CAD build for the part. Positions are in the model's coordinates, mm. A direction names the side the tool comes from. Coordinates: 2 decimals unless noted, no trailing zeros. Loops run counter-clockwise (first coordinate to the right, second up) from the corner with the lowest first, then second, coordinate; pieces in that order, holes last. Notation, with made-up numbers: (25.5, -33.5) -> (66.5, -33.5) arc R29 cw to (66.5, -3.5) -> close; hole circle Ø1 at (33.5, 13.25). An arc over 180 degrees is marked (long way). Write each question's results on one line, items separated by ' | '.
from build123d import *

# Parameters (mm, degrees)
BOSS_EXTRUDE1_DEPTH   = 1.5875
F_4_CLEARANCE_HOLE1_D = 2.9464


with BuildPart() as part:
    # Sketch2 → Boss-Extrude1 (new body)
    with BuildSketch(Plane.XY):
        Polygon((-2.1971, 2.8575), (2.1971, 2.8575), (2.1971, -2.8575), (7.9375, -2.8575), (7.9375, 6.6675), (-7.9375, 6.6675), (-7.9375, -2.8575), (-2.1971, -2.8575), align=None)
    extrude(amount=BOSS_EXTRUDE1_DEPTH)

    # #4 Clearance Hole1 (through all)
    with Locations(Plane.XY.offset(1.5875)):
        with Locations((-5.0673, 1.905), (5.0673, 1.905)):
            Hole(F_4_CLEARANCE_HOLE1_D / 2)


solid = part.part
1) Two-plate mould, pull along X, no slides. Class faces 1 (the cylindrical face through (6.54, 1.97, 0.78)), 2 (the flat face through (-7.938, 2, 1)), 3 (the flat face through (7.938, 2, 1)), 4 (the flat face through (5, -2.858, 1)): pulls with the +X half, pulls with the -X half, needs draft (parallel to the pull), parting line crosses it, or undercut.
Outcome:
face 1: undercut | face 2: pulls with the -X half | face 3: pulls with the +X half | face 4: needs draft
2) Slice it at A-A (y = -2). Write the cut outline in (x, z), then the cut area to 3 significant figures.
Outcome:
outline: (-7.94, 0) -> (-2.2, 0) -> (-2.2, 1.59) -> (-7.94, 1.59) -> close; (2.2, 0) -> (7.94, 0) -> (7.94, 1.59) -> (2.2, 1.59) -> close | area: 18.2 mm^2
3) Which spindle directions (+Z, -Z, +X, -X, +Y, -Y) get a long thin tool onto all of the face, cutting with end or side? Do faces 5 (the flat face through (-0.11, 3.03, 0)), 6 (the flat face through (-2.197, 0, 1)). Say none if no direction does.
Outcome:
face 5: -Z, +X, -X, +Y, -Y | face 6: +Z, -Z, -Y
4) Slice it at C-C (y = 1.25). Write the cut outline in (x, z).
Outcome:
outline: (-7.94, 0) -> (-6.39, 0) -> (-6.39, 1.59) -> (-7.94, 1.59) -> close; (-3.75, 0) -> (-2.2, 0) -> (-2.2, 1.59) -> (-3.75, 1.59) -> close; (2.2, 0) -> (3.75, 0) -> (3.75, 1.59) -> (2.2, 1.59) -> close; (6.39, 0) -> (7.94, 0) -> (7.94, 1.59) -> (6.39, 1.59) -> close
5) Pin check, flat tip, straight feed: pin 1 (1.8 mm diameter, centred on x = 5.07, y = 1.9, fed in from -Z) (1 decimal). Stop position of the tip, or through.
Outcome:
pin 1: passes through
6) Slice it at B-B (x = -5.5). Write the cut outline in (y, z), then the cut area to 3 significant figures.
Outcome:
outline: (-2.86, 0) -> (0.5, 0) -> (0.5, 1.59) -> (-2.86, 1.59) -> close; (3.31, 0) -> (6.67, 0) -> (6.67, 1.59) -> (3.31, 1.59) -> close | area: 10.6 mm^2
7) Drill centre lines: L1, parallel to X at y = 2, z = 0.2; L2, parallel to X at y = 1, z = 0.35; L3, parallel to X at y = -2, z = 1.15. Where is each one in solid material? Low to high. Write a range as from..to.
Outcome:
L1: x = -7.94..-6.54, -3.6..-2.2, 2.2..3.6, 6.54..7.94 | L2: x = -7.94..-6.23, -3.9..-2.2, 2.2..3.9, 6.23..7.94 | L3: x = -7.94..-2.2, 2.2..7.94
8) Slice it at D-D (z = 0.6). Write the cut outline in (x, y) (1 decimal), then the cut area to 3 significant figures.
Outcome:
outline: (-7.9, -2.9) -> (-2.2, -2.9) -> (-2.2, 2.9) -> (2.2, 2.9) -> (2.2, -2.9) -> (7.9, -2.9) -> (7.9, 6.7) -> (-7.9, 6.7) -> close; hole circle Ø2.9 at (-5.1, 1.9); hole circle Ø2.9 at (5.1, 1.9) | area: 112 mm^2
